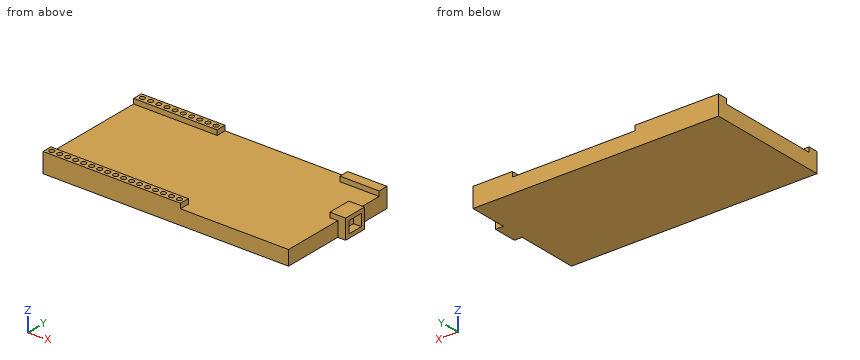
from build123d import *

# Parameters (mm, degrees)
SKETCH1_W           = 125
SKETCH1_H           = 250
BOSS_EXTRUDE1_DEPTH = 15
SKETCH2_W           = 85
SKETCH2_H           = 10
SKETCH2_R           = 2.5
SKETCH2_W_2         = 140
SKETCH2_W_3         = 40
BOSS_EXTRUDE2_DEPTH = 5
SKETCH3_W           = 24
SKETCH3_H           = 20
SKETCH3_W_2         = 16
SKETCH3_H_2         = 12
BOSS_EXTRUDE3_DEPTH = 8
SKETCH4_W           = 24
SKETCH4_H           = 20
BOSS_EXTRUDE4_DEPTH = 8


with BuildPart() as part:
    # Sketch1 → Boss-Extrude1 (new body)
    with BuildSketch(Plane(origin=(0, 0, 0), x_dir=(0, 1, 0), z_dir=(0, 0, 1))):
        Rectangle(SKETCH1_W, SKETCH1_H)
    extrude(amount=BOSS_EXTRUDE1_DEPTH)

    # Sketch2 → Boss-Extrude2 (add)
    # profile 1 of 3: a face of its own
    with BuildSketch(Plane.XY.offset(15)):
        with Locations((-82.5, 57.5)):
            Rectangle(SKETCH2_W, SKETCH2_H)
        with Locations((-120, 57.5)):
            Circle(SKETCH2_R, mode=Mode.SUBTRACT)
        with Locations((-111.666666667, 57.5)):
            Circle(SKETCH2_R, mode=Mode.SUBTRACT)
        with Locations((-103.333333333, 57.5)):
            Circle(SKETCH2_R, mode=Mode.SUBTRACT)
        with Locations((-95, 57.5)):
            Circle(SKETCH2_R, mode=Mode.SUBTRACT)
        with Locations((-86.666666667, 57.5)):
            Circle(SKETCH2_R, mode=Mode.SUBTRACT)
        with Locations((-78.333333333, 57.5)):
            Circle(SKETCH2_R, mode=Mode.SUBTRACT)
        with Locations((-70, 57.5)):
            Circle(SKETCH2_R, mode=Mode.SUBTRACT)
        with Locations((-61.666666667, 57.5)):
            Circle(SKETCH2_R, mode=Mode.SUBTRACT)
        with Locations((-53.333333333, 57.5)):
            Circle(SKETCH2_R, mode=Mode.SUBTRACT)
        with Locations((-45, 57.5)):
            Circle(SKETCH2_R, mode=Mode.SUBTRACT)
    # profile 2 of 3: a face of its own
    with BuildSketch(Plane.XY.offset(15)):
        with Locations((-55, -57.5)):
            Rectangle(SKETCH2_W_2, SKETCH2_H)
        with Locations((-120, -57.5)):
            Circle(SKETCH2_R, mode=Mode.SUBTRACT)
        with Locations((-111.875, -57.5)):
            Circle(SKETCH2_R, mode=Mode.SUBTRACT)
        with Locations((-103.75, -57.5)):
            Circle(SKETCH2_R, mode=Mode.SUBTRACT)
        with Locations((-95.625, -57.5)):
            Circle(SKETCH2_R, mode=Mode.SUBTRACT)
        with Locations((-87.5, -57.5)):
            Circle(SKETCH2_R, mode=Mode.SUBTRACT)
        with Locations((-79.375, -57.5)):
            Circle(SKETCH2_R, mode=Mode.SUBTRACT)
        with Locations((-71.25, -57.5)):
            Circle(SKETCH2_R, mode=Mode.SUBTRACT)
        with Locations((-63.125, -57.5)):
            Circle(SKETCH2_R, mode=Mode.SUBTRACT)
        with Locations((-55, -57.5)):
            Circle(SKETCH2_R, mode=Mode.SUBTRACT)
        with Locations((-46.875, -57.5)):
            Circle(SKETCH2_R, mode=Mode.SUBTRACT)
        with Locations((-38.75, -57.5)):
            Circle(SKETCH2_R, mode=Mode.SUBTRACT)
        with Locations((-30.625, -57.5)):
            Circle(SKETCH2_R, mode=Mode.SUBTRACT)
        with Locations((-22.5, -57.5)):
            Circle(SKETCH2_R, mode=Mode.SUBTRACT)
        with Locations((-14.375, -57.5)):
            Circle(SKETCH2_R, mode=Mode.SUBTRACT)
        with Locations((-6.25, -57.5)):
            Circle(SKETCH2_R, mode=Mode.SUBTRACT)
        with Locations((1.875, -57.5)):
            Circle(SKETCH2_R, mode=Mode.SUBTRACT)
        with Locations((10, -57.5)):
            Circle(SKETCH2_R, mode=Mode.SUBTRACT)
    # profile 3 of 3: a face of its own
    with BuildSketch(Plane.XY.offset(15)):
        with Locations((105, 57.5)):
            Rectangle(SKETCH2_W_3, SKETCH2_H)
    extrude(amount=BOSS_EXTRUDE2_DEPTH)

    # Sketch3 → Boss-Extrude3 (add)
    with BuildSketch(Plane.YZ.offset(125)):
        with Locations((12, 10)):
            Rectangle(SKETCH3_W, SKETCH3_H)
        with Locations((12, 10)):
            Rectangle(SKETCH3_W_2, SKETCH3_H_2, mode=Mode.SUBTRACT)
    extrude(amount=BOSS_EXTRUDE3_DEPTH)

    # Sketch4 → Boss-Extrude4 (add)
    with BuildSketch(Plane(origin=(125, 0, 0), x_dir=(0, -1, 0), z_dir=(-1, 0, 0))):
        with Locations((-12, 10)):
            Rectangle(SKETCH4_W, SKETCH4_H)
    extrude(amount=BOSS_EXTRUDE4_DEPTH)


solid = part.part
Geometry: final body of the model. Coordinates: model frame, mm. Give positions to 0.01 mm unless a question says otherwise; leave off trailing zeros. Write each loop counter-clockwise with the first axis right and the second up, starting at its lowest first coordinate (ties: lowest second). Pieces come first, ordered by that corner, then holes. Notation, with made-up numbers: (1.25, -32.75) - (13.25, -32.75) arc R15 cw to (13.25, -28.75) - close; hole circle Ø11 at (-31, 41). An arc over 180 degrees is marked (long way). Return JSON: item names as keys, results as strings. Group by question number.
1) Section D-D on y = 39. Return the cut outline in (x, z), plus the area to 3 significant figures.
2) Section B-B on z = 6.5. Return the cut outline in (x, y).
3) Section C-C on x = 90. Return the cut outline in (y, z), plus the area to 4 significant figures.
4) Line query: line 1 (Y direction, x = -42, z = 18.5); line 2 (Y direction, x = -103.75, z = 16.1); line 3 (Z direction, x = -81, y = 46). Output: solid intervals per line, ascending.
5) Section A-A on x = -22.5. Return the cut outline in (y, z).
6) First-contact query: P1, Ø12, axis at x = 59, y = 31.5, coming from the +Z side; P2, Ø3.5, axis at y = 10.5, z = 11, coming from the +X side. Flat tips, straight axial feed; report the tip coordinate or a pass-through.
Filled in:
{
 "1": {"outline": "(-125, 0) - (125, 0) - (125, 15) - (-125, 15) - close", "area": "3,750 mm^2"},
 "2": {"outline": "(-125, -62.5) - (125, -62.5) - (125, 0) - (133, 0) - (133, 4) - (125, 4) - (125, 20) - (133, 20) - (133, 24) - (125, 24) - (125, 62.5) - (-125, 62.5) - close"},
 "3": {"outline": "(-62.5, 0) - (62.5, 0) - (62.5, 20) - (52.5, 20) - (52.5, 15) - (-62.5, 15) - close", "area": "1,925 mm^2"},
 "4": {"line 1": "y = -62.5 to -52.5, 52.5 to 62.5", "line 2": "y = -62.5 to -60, -55 to -52.5, 52.5 to 55.03, 59.97 to 62.5", "line 3": "z = 0 to 15"},
 "5": {"outline": "(-62.5, 0) - (62.5, 0) - (62.5, 15) - (-52.5, 15) - (-52.5, 20) - (-55, 20) - (-55, 15) - (-60, 15) - (-60, 20) - (-62.5, 20) - close"},
 "6": {"P1": "stops at z = 15", "P2": "stops at x = 125"}
}
